```python
from build123d import *

# Parameters (mm, degrees)
SKETCH1_W           = 25.4
SKETCH1_H           = 25.4
SKETCH1_W_2         = 20.32
SKETCH1_H_2         = 20.32
BOSS_EXTRUDE1_DEPTH = 127
SKETCH2_W           = 25.4
SKETCH2_H           = 12.7
CUT_EXTRUDE1_DEPTH  = 127
FILLET1_R           = 25.4
SKETCH3_R           = 3.175
CUT_EXTRUDE2_DEPTH  = 127
SKETCH4_R           = 9.525
CUT_EXTRUDE3_DEPTH  = 127
CUT_EXTRUDE4_DEPTH  = 127


with BuildPart() as part:
    # Sketch1 → Boss-Extrude1 (new body)
    with BuildSketch(Plane(origin=(0, 0, 0), x_dir=(0, 0, -1), z_dir=(1, 0, 0))):
        with Locations((12.7, 12.7)):
            Rectangle(SKETCH1_W, SKETCH1_H)
        with Locations((12.7, 12.7)):
            Rectangle(SKETCH1_W_2, SKETCH1_H_2, mode=Mode.SUBTRACT)
    extrude(amount=BOSS_EXTRUDE1_DEPTH)

    # Sketch2 → Cut-Extrude1 (cut)
    with BuildSketch(Plane.XY):
        with Locations((63.5, 19.05)):
            Rectangle(SKETCH2_W, SKETCH2_H)
    extrude(amount=-CUT_EXTRUDE1_DEPTH, mode=Mode.SUBTRACT)

    # Fillet1
    # the kernel refuses this fillet: 25.4 mm, written as the material it takes off along each edge
    with BuildSketch(Plane(origin=(0, 25.4, -88.9), x_dir=(0, -1, 0), z_dir=(0, 0, 1))) as fillet1_piece_1:
        with BuildLine():
            CenterArc((FILLET1_R, FILLET1_R), FILLET1_R, 180, 90)
            Line((0, FILLET1_R), (0, 0))
            Line((0, 0), (FILLET1_R, 0))
        make_face()
    extrude(amount=152.4, mode=Mode.SUBTRACT)

    # Sketch3 → Cut-Extrude2 (cut)
    with BuildSketch(Plane.XY):
        with Locations((7.62, 7.62)):
            Circle(SKETCH3_R)
        with Locations((17.78, 17.78)):
            Circle(SKETCH3_R)
    extrude(amount=-CUT_EXTRUDE2_DEPTH, mode=Mode.SUBTRACT)

    # Sketch4 → Cut-Extrude3 (cut)
    with BuildSketch(Plane.XY):
        with Locations((107.95, 12.7)):
            Circle(SKETCH4_R)
    extrude(amount=-CUT_EXTRUDE3_DEPTH, mode=Mode.SUBTRACT)

    # Sketch5 → Cut-Extrude4 (cut)
    with BuildSketch(Plane.XZ):
        with BuildLine():
            Line((91.44, -3.81), (93.98, -3.81))
            ThreePointArc((93.98, -3.81), (94.878025612, -4.181974388), (95.25, -5.08))
            Line((95.25, -5.08), (95.25, -20.32))
            ThreePointArc((95.25, -20.32), (94.878025612, -21.218025612), (93.98, -21.59))
            Line((93.98, -21.59), (91.44, -21.59))
            ThreePointArc((91.44, -21.59), (90.541974388, -21.218025612), (90.17, -20.32))
            Line((90.17, -20.32), (90.17, -5.08))
            ThreePointArc((90.17, -5.08), (90.541974388, -4.181974388), (91.44, -3.81))
        make_face()
    extrude(amount=-CUT_EXTRUDE4_DEPTH, mode=Mode.SUBTRACT)


solid = part.part
```
Could you check a few things on this model? Use its own coordinates, in mm. A direction names the side the tool comes from. Coordinates: 2 decimals unless noted, no trailing zeros. Write each loop counter-clockwise with the first axis right and the second up, starting at its lowest first coordinate (ties: lowest second). Pieces come first, ordered by that corner, then holes. Notation, with made-up numbers: (47.5, 65.5) -> (100.5, 65.5) arc R25 ccw to (100.5, 90.5) -> close; hole circle Ø10 at (-35, 89). An arc over 180 degrees is marked (long way). Return JSON: item names as keys, results as strings.
(1) Imagine slicing it at A-A, the plane x = 107.95. Please give me the cut outline in (y, z) (3 decimals).
Numbers:
{"outline": "(0, -25.4) -> (3.175, -25.4) -> (3.175, -22.86) -> (2.54, -22.86) -> (2.54, -2.54) -> (3.175, -2.54) -> (3.175, 0) -> (0, 0) -> close; (22.225, -25.4) -> (25.4, -25.4) -> (25.4, 0) -> (22.225, 0) -> (22.225, -2.54) -> (22.86, -2.54) -> (22.86, -22.86) -> (22.225, -22.86) -> close"}
(2) I need wall thicknesses on L1, parallel to Z at x = 81.5, y = 19.75; L2, parallel to Y at x = 99, z = -8.5; L3, parallel to Y at x = 107.95, z = -24.7 (3 decimals). Which ranges of each line are inside material? Lowest first, please.
Numbers:
{"L1": "z = -25.4 to -22.86, -2.54 to 0", "L2": "y = 0 to 2.54, 22.86 to 25.4", "L3": "y = 0 to 3.175, 22.225 to 25.4"}
(3) Which directions (+Z, -Z, +X, -X, +Y, -Y) give clear straight access to the entire face, cutting with the end or side of a thin tool? Please do faces 1 (the flat face through (76.2, 23.2, -12.5)), 2 (the flat face through (63, 10, -22.86)), 3 (the flat face through (93, 24, -21.59)).
Numbers:
{"face 1": "+Z, -Z, +Y", "face 2": "+X, -X", "face 3": "+Y, -Y"}
(4) I'm going to push flat-ended pins straight in: pin 1 (10 mm diameter, centred on x = 17.78, y = 17.78, fed in from +Z); pin 2 (3 mm diameter, centred on y = 6, z = -9, fed in from -X); pin 3 (2 mm diameter, centred on x = 57.5, z = -13.5, fed in from +Y); pin 4 (6.5 mm diameter, centred on y = 20.5, z = -10.5, fed in from -X). Where does each tip first touch, or does it pass through?
Numbers:
{"pin 1": "stops at z = 0", "pin 2": "passes through", "pin 3": "stops at y = 2.54", "pin 4": "stops at x = 14.33"}
(5) Imagine slicing it at C-C, the plane z = -9.75. Please give me the cut outline in (x, y), then the cut area to 3 significant figures.
Numbers:
{"outline": "(0, 0) -> (90.17, 0) -> (90.17, 2.54) -> (0.13, 2.54) arc R25.4 ccw to start; (14.33, 22.86) -> (50.8, 22.86) -> (50.8, 25.4) -> (25.4, 25.4) arc R25.4 ccw to start; (76.2, 22.86) -> (90.17, 22.86) -> (90.17, 25.4) -> (76.2, 25.4) -> close; (95.25, 0) -> (127, 0) -> (127, 2.54) -> (95.25, 2.54) -> close; (95.25, 22.86) -> (127, 22.86) -> (127, 25.4) -> (95.25, 25.4) -> close", "area": "509 mm2"}
(6) We'd pull the mould along Z, two halves only. Please class faces 4 (the flat face through (32, 22.86, -13)), 5 (the flat face through (63, 0, -13)), 6 (the flat face through (62.6, 12.5, 0)): +Z half, -Z half, draft (parallel to the pull), parting line (faces both ways), or undercut.
Numbers:
{"face 4": "undercut", "face 5": "draft", "face 6": "+Z half"}
(7) Imagine slicing it at B-B, the plane x = 88. Please give me the cut outline in (y, z).
Numbers:
{"outline": "(0, -25.4) -> (25.4, -25.4) -> (25.4, 0) -> (0, 0) -> close; hole (2.54, -22.86) -> (22.86, -22.86) -> (22.86, -2.54) -> (2.54, -2.54) -> close"}
(8) Imagine slicing it at D-D, the plane y = 16.25. Count the separate pieces of the cut face and the enclosed holes in it, then the cut area to 3 significant figures.
Numbers:
{"separate pieces": "8", "enclosed holes": "0", "area": "368 mm2"}
